```python
from build123d import *

# Parameters (mm, degrees)
F0_W     = 251.524948
F0_H     = 283.958055
F0_R     = 1.7272
F0_W_2   = 9.525
F0_H_2   = 9.525
F0_R_2   = 3.175
F0_W_3   = 40.64
F0_H_3   = 19.558
F1_DEPTH = 5.08


with BuildPart() as f1:
    # F0 (on Top) → F1 (new body)
    with BuildSketch(Plane.XY):
        with Locations((125.762474, -141.979028)):
            Rectangle(F0_W, F0_H)
        with Locations((4.7625, -279.195555)):
            Circle(F0_R, mode=Mode.SUBTRACT)
        with Locations((60.325, -279.195555)):
            Circle(F0_R, mode=Mode.SUBTRACT)
        with Locations((92.9275, -269.670555)):
            Rectangle(F0_W_2, F0_H_2, mode=Mode.SUBTRACT)
        with Locations((125.762474, -215.9)):
            Circle(F0_R_2, mode=Mode.SUBTRACT)
        with Locations((134.362469, -269.670555)):
            Rectangle(F0_W_2, F0_H_2, mode=Mode.SUBTRACT)
        with Locations((125.762474, -253.541555)):
            Rectangle(F0_W_3, F0_H_3, mode=Mode.SUBTRACT)
        with Locations((167.197443, -269.670555)):
            Rectangle(F0_W_2, F0_H_2, mode=Mode.SUBTRACT)
        with Locations((191.199948, -279.195555)):
            Circle(F0_R, mode=Mode.SUBTRACT)
        with Locations((246.762448, -279.195555)):
            Circle(F0_R, mode=Mode.SUBTRACT)
        with Locations((37.774293, -63.5)):
            Circle(F0_R_2, mode=Mode.SUBTRACT)
        with Locations((4.7625, -4.7625)):
            Circle(F0_R, mode=Mode.SUBTRACT)
        with Locations((60.325, -4.7625)):
            Circle(F0_R, mode=Mode.SUBTRACT)
        with Locations((92.9275, -14.2875)):
            Rectangle(F0_W_2, F0_H_2, mode=Mode.SUBTRACT)
        with Locations((92.9275, -4.7625)):
            Circle(F0_R, mode=Mode.SUBTRACT)
        with Locations((134.362469, -14.2875)):
            Rectangle(F0_W_2, F0_H_2, mode=Mode.SUBTRACT)
        with Locations((134.362469, -4.7625)):
            Circle(F0_R, mode=Mode.SUBTRACT)
        with Locations((167.197443, -14.2875)):
            Rectangle(F0_W_2, F0_H_2, mode=Mode.SUBTRACT)
        with Locations((167.197443, -4.7625)):
            Circle(F0_R, mode=Mode.SUBTRACT)
        with Locations((213.750655, -63.5)):
            Circle(F0_R_2, mode=Mode.SUBTRACT)
        with Locations((191.199948, -4.7625)):
            Circle(F0_R, mode=Mode.SUBTRACT)
        with Locations((246.762448, -4.7625)):
            Circle(F0_R, mode=Mode.SUBTRACT)
    extrude(amount=F1_DEPTH)


solid = f1.part
```
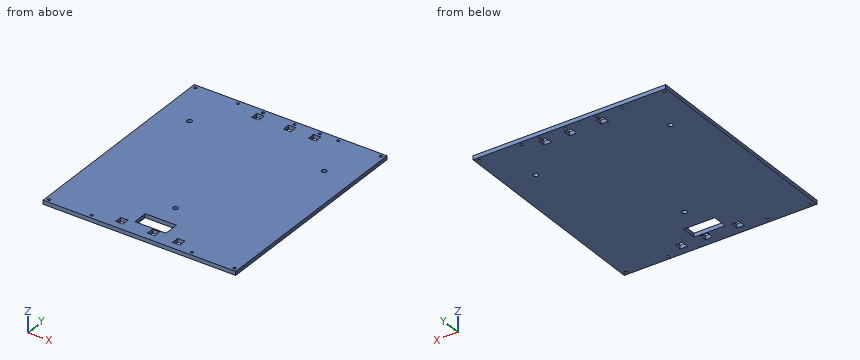
Could you check a few things on this model? Use its own coordinates, in mm. Coordinates: 2 decimals unless noted, no trailing zeros. Order: outer loops, then holes, each group sorted by start corner. A loop starts at its lowest first (then second) coordinate and runs counter-clockwise, first axis right, second up. Notation, with made-up numbers: M 63.5,-34.75 L 95.5,-34.75 A28 ccw 95.5,-11.75 Z; hole C 28,39 d5. An arc over 180 degrees is marked long. Use one line per item in the form item = value. Start each with the question number.
1. Please list where these lines run through material, in increasing order: line 1 (X direction, y = -245.5, z = 1.7); line 2 (Y direction, x = 162.5, z = 3.7) (3 decimals); line 3 (X direction, y = -215.9, z = 3.8).
2. Suppose I cut it at B-B on y = -215.9. Write out the boundary of the cut face in (x, z).
3. Suppose I cut it at A-A on y = -63.5. Write out the boundary of the cut face in (x, z).
4. Suppose I cut it at C-C on z = 2.45. Count the separate pieces of the cut face and the enclosed holes in it, then the cut area to 3 significant figures.
Geometry says:
q1.line_1 = 0 to 105.44, 146.08 to 251.52
q1.line_2 = -283.958 to -274.433, -264.908 to -19.05, -9.525 to 0
q1.line_3 = 0 to 122.59, 128.94 to 251.52
q2.outline = M 0,0 L 122.59,0 L 122.59,5.08 L 0,5.08 Z; M 128.94,0 L 251.52,0 L 251.52,5.08 L 128.94,5.08 Z
q3.outline = M 0,0 L 34.6,0 L 34.6,5.08 L 0,5.08 Z; M 40.95,0 L 210.58,0 L 210.58,5.08 L 40.95,5.08 Z; M 216.93,0 L 251.52,0 L 251.52,5.08 L 216.93,5.08 Z
q4.separate_pieces = 1
q4.enclosed_holes = 21
q4.area = 69,900 mm^2
